from build123d import *

# Parameters (mm, degrees)
SCHIZZO1_R                   = 6.5
ESTRUSIONE_ESTRUSIONE1_DEPTH = 14
SCHIZZO2_R                   = 6
ESTRUSIONE_ESTRUSIONE2_DEPTH = 13
CUPOLA1_FACE_RADIUS          = 6
CUPOLA1_HEIGHT               = 5.61
ESTRUSIONE_ESTRUSIONE3_DEPTH = 7.5
RACCORDO1_R                  = 2


with BuildPart() as part:
    # Schizzo1 → Estrusione-Estrusione1 (new body)
    with BuildSketch(Plane.XY):
        Circle(SCHIZZO1_R)
    extrude(amount=ESTRUSIONE_ESTRUSIONE1_DEPTH)

    # Schizzo2 → Estrusione-Estrusione2 (add)
    with BuildSketch(Plane.XY.offset(14)):
        with Locations(Location((0, 0, 0), (0, 0, 180))):
            Circle(SCHIZZO2_R)
    extrude(amount=ESTRUSIONE_ESTRUSIONE2_DEPTH)

    # Cupola1: a dome of height H over a round flat face of radius A is a cap of a sphere of radius (A * A + H * H) / (2 * H)
    cupola1_r = (CUPOLA1_FACE_RADIUS * CUPOLA1_FACE_RADIUS + CUPOLA1_HEIGHT * CUPOLA1_HEIGHT) / (2 * CUPOLA1_HEIGHT)
    cupola1_base = Plane((0, 0, 27), z_dir=(0, 0, 1))
    with Locations(cupola1_base.offset(CUPOLA1_HEIGHT - cupola1_r)):
        cupola1_ball = Sphere(cupola1_r, mode=Mode.PRIVATE)
    add(split(cupola1_ball, bisect_by=cupola1_base, keep=Keep.TOP, mode=Mode.PRIVATE))

    # Schizzo3 → Estrusione-Estrusione3 (add, symmetric)
    with BuildSketch(Plane(origin=(0, 0, 0), x_dir=(1, 0, 0), z_dir=(0, 1, 0))):
        with BuildLine():
            Line((-6.5, 2), (-6.5, 0))
            Line((-6.5, 0), (0, 0))
            Line((0, 0), (0, 28.411501065))
            Line((0, 28.411501065), (-5.385587173, 19.792759953))
            ThreePointArc((-5.385587173, 19.792759953), (-9.163389911, 11.254561696), (-10.398586576, 2))
            Line((-10.398586576, 2), (-6.5, 2))
        make_face()
        with BuildLine():
            Line((0, 28.411501065), (0, 0))
            Line((0, 0), (6.5, 0))
            Line((6.5, 0), (6.5, 2))
            Line((6.5, 2), (10.401413424, 2))
            ThreePointArc((10.401413424, 2), (13.142849654, 15.477548319), (21.139966273, 26.667092863))
            ThreePointArc((21.139966273, 26.667092863), (19.525120405, 78.287820261), (-24.93, 52))
            Line((-24.93, 52), (-24.335940594, 46.059405941))
            Line((-24.335940594, 46.059405941), (-23.43, 37))
            ThreePointArc((-23.43, 37), (-18.43, 32), (-13.43, 37))
            Line((-13.43, 37), (-12.5, 52))
            ThreePointArc((-12.5, 52), (3.445466948, 64.015771199), (10.600601202, 45.376009197))
            Line((10.600601202, 45.376009197), (0, 28.411501065))
        make_face()
    extrude(amount=ESTRUSIONE_ESTRUSIONE3_DEPTH, both=True)

    # Raccordo1
    raccordo1_edges = [part.edges().sort_by_distance(p)[0] for p in [
        (6.5, 0, -2),
        (-6.5, 0, -2),
    ]]
    fillet(raccordo1_edges, radius=RACCORDO1_R - 0.0001)  # a hair under: the kernel refuses the full size


solid = part.part
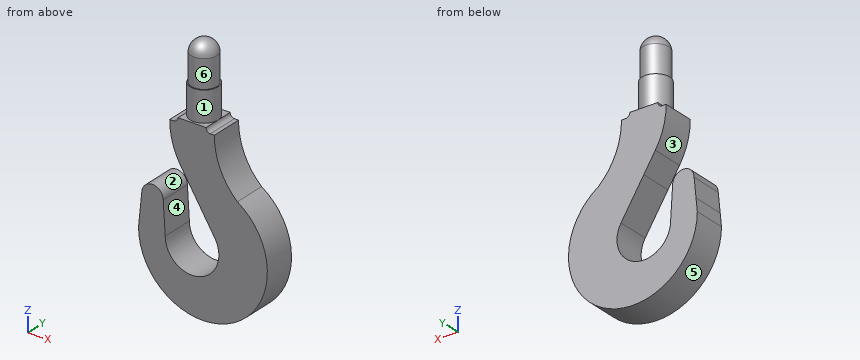
Here's how the part is built. I have some questions about the finished solid (model axes, mm). Face numbers are marked on the shaded views. A direction names the side the tool comes from. Coordinates: 2 decimals unless noted, no trailing zeros. Loops run counter-clockwise (first coordinate to the right, second up) from the corner with the lowest first, then second, coordinate; pieces in that order, holes last.
1. If we mould it in two halves opening along Z, with no side actions, what happens to the marked faces 1, 2 and 3? For each: pulls with the +Z half, pulls with the -Z half, needs draft (parallel to the pull), parting line crosses it, or undercut.
2. I need wall thicknesses on L1, parallel to X at y = -4, z = -52; L2, parallel to Z at x = 0, y = 3.25; L3, parallel to Z at x = 0, y = 1. Which ranges of each line are inside material? Lowest first, please.
3. Imagine slicing it at A-A, the plane z = -61.5. Please give me the cut outline in (x, y).
4. Imagine slicing it at D-D, the plane x = 20. Please give me the cut outline in (y, z), and give its area (3 significant figures).
5. For P1, Ø4, axis at x = 16.5, y = -6, coming from the -Z side; P2, Ø0.6, axis at x = -9.5, y = 2.5, coming from the +Z side; P3, Ø2.5, axis at x = -1.5, y = 4.5, coming from the +Z side; P4, Ø20, axis at x = 0, z = -52, coming from the -Y side, each with a flat end and sliding along its axis, tell me the tip position at first contact or that it passes through.
6. Imagine slicing it at C-C, the plane z = 2.5. Please give me the cut outline in (x, y), and give its area (3 significant figures).
7. For the marked faces 4, 5 and 6, which set-ups out of +Z, -Z, +X, -X, +Y, -Y let a thin tool reach every point of the face, with its end or its side?
Taken from the geometry:
1. face 1: needs draft
1. face 2: pulls with the +Z half
1. face 3: undercut
2. L1: x = -24.93 to -12.5, 12.5 to 35.07
2. L2: z = -81.57 to -64.5, -28.41 to 31.66
2. L3: z = -81.57 to -64.5, -28.41 to 32.53
3. outline: (-23.39, -7.5) - (-8.12, -7.5) - (-8.12, 7.5) - (-23.39, 7.5) - close; (8.12, -7.5) - (33.53, -7.5) - (33.53, 7.5) - (8.12, 7.5) - close
4. outline: (-7.5, -78.02) - (7.5, -78.02) - (7.5, -25.57) - (-7.5, -25.57) - close
4. area: 787 mm2
5. P1: stops at z = -80.48
5. P2: stops at z = -2
5. P3: stops at z = 31.49
5. P4: passes through
6. outline: circle Ø13 at (0, 0)
6. area: 133 mm2
7. face 4: +Z, +Y, -Y
7. face 5: +Y, -Y
7. face 6: +Z
